Drawing for the job (mm, zero at the part's lowest x, y, z). A direction names the side the tool comes from. Round coordinates to 2 decimals unless told otherwise and drop trailing zeros. Write each loop counter-clockwise with the first axis right and the second up, starting at its lowest first coordinate (ties: lowest second). Pieces come first, ordered by that corner, then holes.
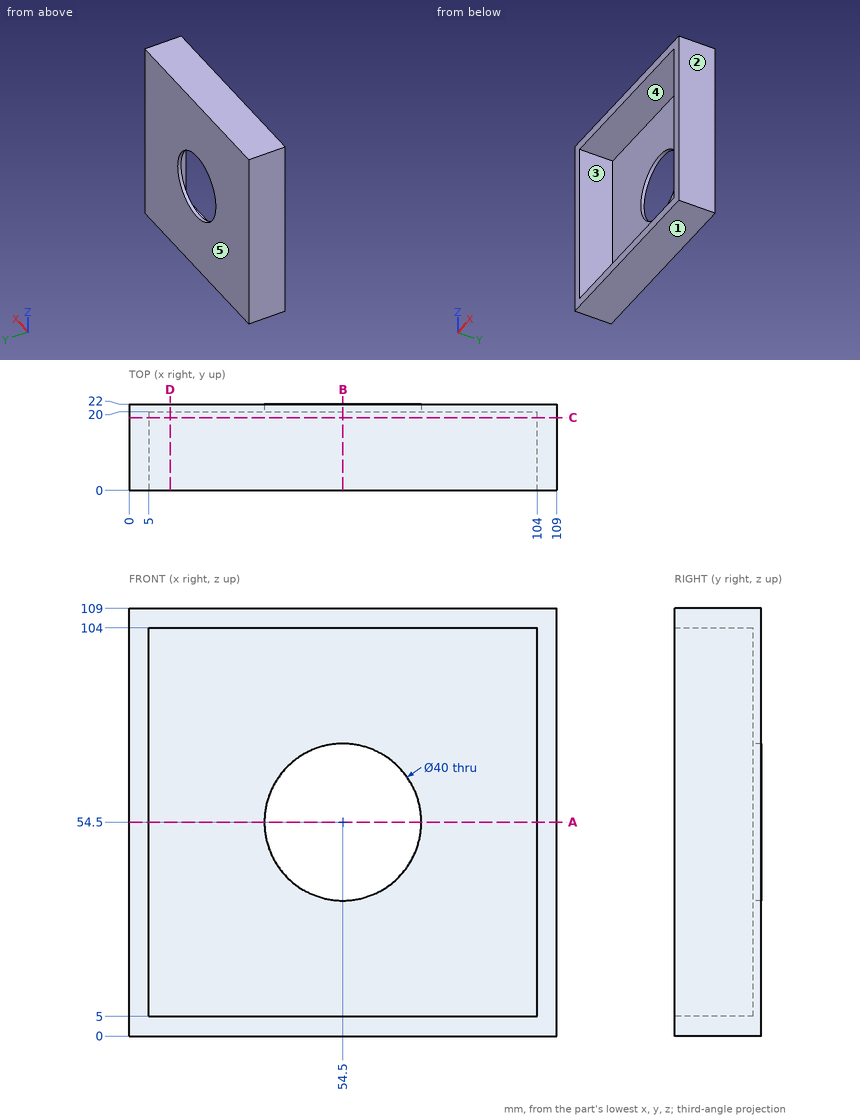
1) Flat gauge pins, fed straight in: pin 1 Ø6 at (x, y) = (54.5, 9) entering from -Z; pin 2 Ø3 at (x, z) = (72, 13) entering from -Y. Where does each tip first touch, or does it go through?
2) Cut at C-C on y = 18.5. List the corners of the cut face in (x, z).
3) Cut at A-A on z = 54.5. List the corners of the cut face in (x, y), and give its area (3 significant figures).
4) Pull direction Z, two halves, no side cores. Call the marked faces 1, 2 and 3: released by +Z, released by -Z, zero draft, split by the parting line, or undercut.
5) Which spindle directions (+Z, -Z, +X, -X, +Y, -Y) get a long thin tool onto all of the face, cutting with end or side? Do the marked faces 4 and 5. Say none if no direction does.
6) Wall check: probe 1 along Z at (x, y) = (73.5, 16.75); probe 2 along Z at (x, y) = (54.5, 20.6). Give the ranges that are in metal, low to high.
7) Cut at B-B on x = 54.5. List the corners of the cut face in (y, z), and give its area (3 significant figures).
8) Cut at D-D on x = 10.5. List the corners of the cut face in (y, z).
Result sheet:
1. pin 1: stops at z = 0
1. pin 2: stops at y = 20
2. outline: (0, 0) - (109, 0) - (109, 109) - (0, 109) - close; hole (5, 5) - (104, 5) - (104, 104) - (5, 104) - close
3. outline: (0, 0) - (5, 0) - (5, 20) - (34.5, 20) - (34.5, 22) - (0, 22) - close; (74.5, 20) - (104, 20) - (104, 0) - (109, 0) - (109, 22) - (74.5, 22) - close
3. area: 338 mm2
4. face 1: released by -Z
4. face 2: zero draft
4. face 3: undercut
5. face 4: -Y
5. face 5: +Z, -Z, +X, -X, +Y
6. probe 1: z = 0 to 5, 104 to 109
6. probe 2: z = 0 to 34.5, 74.5 to 109
7. outline: (0, 0) - (22, 0) - (22, 34.5) - (20, 34.5) - (20, 5) - (0, 5) - close; (0, 104) - (20, 104) - (20, 74.5) - (22, 74.5) - (22, 109) - (0, 109) - close
7. area: 338 mm2
8. outline: (0, 0) - (22, 0) - (22, 109) - (0, 109) - (0, 104) - (20, 104) - (20, 5) - (0, 5) - close
